```python
from build123d import *
from OCP.BRepFilletAPI import BRepFilletAPI_MakeChamfer

# Parameters (mm, degrees)
SCHIZZO1_W                   = 900
SCHIZZO1_H                   = 900
ESTRUSIONE_ESTRUSIONE1_DEPTH = 31.5
SMUSSO1_SIZE                 = 100
SMUSSO1_SIZE2                = 173.205080757
SMUSSO2_SIZE                 = 100
SMUSSO2_SIZE2                = 173.205080757


with BuildPart() as part:
    # Schizzo1 → Estrusione-Estrusione1 (new body)
    with BuildSketch(Plane.XY):
        Rectangle(SCHIZZO1_W, SCHIZZO1_H)
    extrude(amount=ESTRUSIONE_ESTRUSIONE1_DEPTH)

    # Smusso1: one chamfer whose edges measure the first distance from different faces: ONE call of the kernel's chamfer builder (chamfer() names one face for all edges)
    smusso1_edges_1 = [part.edges().sort_by_distance(p)[0] for p in [
        (450, -450, 15.75),
    ]]
    smusso1_side_1 = [part.faces().sort_by_distance(p)[0] for p in [
        (0, -450, 15.75),
    ]]
    smusso1_edges_2 = [part.edges().sort_by_distance(p)[0] for p in [
        (-450, 450, 15.75),
    ]]
    smusso1_side_2 = [part.faces().sort_by_distance(p)[0] for p in [
        (0, 450, 15.75),
    ]]
    smusso1 = BRepFilletAPI_MakeChamfer(part.part.solid().wrapped)
    for e in smusso1_edges_1:
        smusso1.Add(SMUSSO1_SIZE, SMUSSO1_SIZE2, e.wrapped, smusso1_side_1[0].wrapped)  # the first distance lies on this face
    for e in smusso1_edges_2:
        smusso1.Add(SMUSSO1_SIZE, SMUSSO1_SIZE2, e.wrapped, smusso1_side_2[0].wrapped)  # the first distance lies on this face
    add(Compound.cast(smusso1.Shape()), mode=Mode.REPLACE)

    # Smusso2: one chamfer whose edges measure the first distance from different faces: ONE call of the kernel's chamfer builder (chamfer() names one face for all edges)
    smusso2_edges_1 = [part.edges().sort_by_distance(p)[0] for p in [
        (-450, -450, 15.75),
    ]]
    smusso2_side_1 = [part.faces().sort_by_distance(p)[0] for p in [
        (-50, -450, 15.75),
    ]]
    smusso2_edges_2 = [part.edges().sort_by_distance(p)[0] for p in [
        (450, 450, 15.75),
    ]]
    smusso2_side_2 = [part.faces().sort_by_distance(p)[0] for p in [
        (50, 450, 15.75),
    ]]
    smusso2 = BRepFilletAPI_MakeChamfer(part.part.solid().wrapped)
    for e in smusso2_edges_1:
        smusso2.Add(SMUSSO2_SIZE, SMUSSO2_SIZE2, e.wrapped, smusso2_side_1[0].wrapped)  # the first distance lies on this face
    for e in smusso2_edges_2:
        smusso2.Add(SMUSSO2_SIZE, SMUSSO2_SIZE2, e.wrapped, smusso2_side_2[0].wrapped)  # the first distance lies on this face
    add(Compound.cast(smusso2.Shape()), mode=Mode.REPLACE)


solid = part.part
```
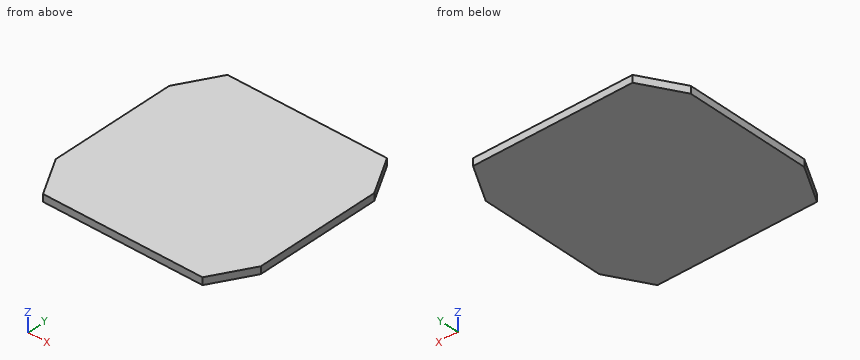
Geometry check sheet. Reference: the model listing, model coordinates, mm. Round coordinates to 2 decimals unless told otherwise and drop trailing zeros. Order: outer loops, then holes, each group sorted by start corner. A loop starts at its lowest first (then second) coordinate and runs counter-clockwise, first axis right, second up. Notation, with made-up numbers: (40, 13) - (52, 13) arc R19 cw to (52, 41) - close; hole circle Ø1 at (-16, 21.5). An arc over 180 degrees is marked (long way). Use a Markdown table: item, result. Add a question column.
1) Gauge pin test, flat end, axial feed: P1, Ø1, axis at y = 310, z = 21.5, coming from the -X side. Record the tip position at first contact, or that the pin passes through.
2) Thickness scan on line 1 along X through (y, z) = (355.5, 18); line 2 along X through (y, z) = (367.5, 30); line 3 along Y through (x, z) = (396.5, 8.5). Record the ranges inside material, lowest first.
3) Section check B-B (x = 373). Record the cut outline in (y, z), then the cut area to 3 significant figures.
4) Section check C-C (y = -303.5). Record the cut outline in (x, z).
5) Section check A-A (z = 17). Record the cut outline in (x, y).
Established:
| question | item | result |
|---|---|---|
| 1 | P1 | x = -431.12 |
| 2 | line 1 | -404.56 to 404.56 |
| 2 | line 2 | -397.63 to 397.63 |
| 2 | line 3 | -369.46 to 369.46 |
| 3 | outline | (-410.16, 0) - (410.16, 0) - (410.16, 31.5) - (-410.16, 31.5) - close |
| 3 | area | 25,800 mm2 |
| 4 | outline | (-434.58, 0) - (434.58, 0) - (434.58, 31.5) - (-434.58, 31.5) - close |
| 5 | outline | (-450, -276.79) - (-350, -450) - (350, -450) - (450, -276.79) - (450, 276.79) - (350, 450) - (-350, 450) - (-450, 276.79) - close |
